Autodesk Inventor part; units mm, degrees
ref_plane "Startebene" through (0, 0, 0) normal (1, 0, 0) x (0, 1, 0)
ref_plane "XZ Plane" through (0, 0, 0) normal (0, 1, 0) x (-1, 0, 0)
ref_plane "XY Plane" through (0, 0, 0) normal (0, 0, 1) x (1, 0, 0)
sketch "Hauptskizze" plane through (0, 0, 0) normal (0, 0, 1) x (1, 0, 0)
  line L0 (0, 0) -> (50, 0)
  line L1 (0, 0) -> (0, 3)
  line L2 (50, 3) -> (50, 0)
  line L3 (0, 3) -> (50, 3)
  dimension "d3" = 6
revolve "Umdrehung1" add sketch "Hauptskizze" angle 360 about axis through (0, 0, 0) along (1, 0, 0)
chamfer "Fase3" distance 0.5 angle 45 1 edges at (0, -3, 0) measured on face at (33.3333, 2.9612, -0.4812)
chamfer "Fase2" distance 0.5 angle 45 1 edges at (50, -3, 0) measured on face at (17, 2.9903, -0.2414)
properties part number "Welle" material "Steel"
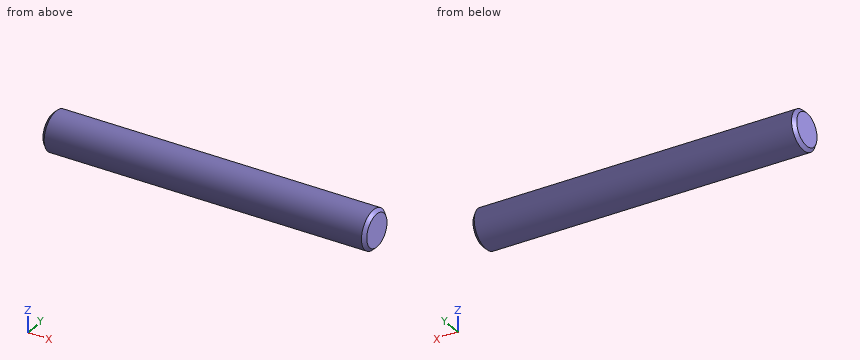
Here's how the part is built. I have some questions about the finished solid (model axes, mm). Coordinates: 2 decimals unless noted, no trailing zeros. Order: outer loops, then holes, each group sorted by start corner. A loop starts at its lowest first (then second) coordinate and runs counter-clockwise, first axis right, second up. Notation, with made-up numbers: (83, 26.25) -> (94, 26.25) arc R19 ccw to (94, 56.25) -> close; hole circle Ø6 at (-14, 25.25). An arc over 180 degrees is marked (long way). Return JSON: item names as keys, results as strings.
1) If I drill on probe 1 along Z at (x, y) = (32.5, 1.65); probe 2 along Z at (x, y) = (32, 0.1); probe 3 along Y at (x, z) = (27.5, -1.95), over which ranges is the centre line in solid material (lowest first)?
Conclusion:
{"probe 1": "z = -2.51 to 2.51", "probe 2": "z = -3 to 3", "probe 3": "y = -2.28 to 2.28"}
2) I'm going to push flat-ended pins straight in: P1, Ø1, axis at y = 1.5, z = 2.5, coming from the +X side; P2, Ø1.5, axis at x = 7.5, y = 1, coming from the +Z side. Where does each tip first touch, or does it pass through?
Conclusion:
{"P1": "stops at x = 50", "P2": "stops at z = 2.99"}
3) If we section it at A-A on x = 41: List the corners of the cut face in (y, z) for me.
Conclusion:
{"outline": "circle Ø6 at (0, 0)"}
